For this review, take the finished solid that the model builds, in its own axes (mm). Coordinates: 2 decimals unless noted, no trailing zeros. Write each loop counter-clockwise with the first axis right and the second up, starting at its lowest first coordinate (ties: lowest second). Pieces come first, ordered by that corner, then holes.
```python
from build123d import *

# Parameters (mm, degrees)
CROQUIS1_R              = 3
CROQUIS1_R_2            = 4
SALIENTE_EXTRUIR1_DEPTH = 3


with BuildPart() as part:
    # Croquis1 → Saliente-Extruir1 (new body)
    with BuildSketch(Plane(origin=(0, 0, 0), x_dir=(1, 0, 0), z_dir=(0, 1, 0))):
        Polygon((17, 27.5), (0, 27.5), (-17, 27.5), (-17, 30.5), (-23.75, 30.5), (-30.5, 30.5), (-30.5, 23.75), (-40.5, 23.75), (-40.5, 8), (-37.5, 8), (-37.5, 0), (-37.5, -8), (-40.5, -8), (-40.5, -23.75), (-30.5, -23.75), (-30.5, -30.5), (-23.75, -30.5), (-17, -30.5), (-17, -27.5), (0, -27.5), (17, -27.5), (17, -30.5), (23.75, -30.5), (30.5, -30.5), (30.5, -23.75), (40.5, -23.75), (40.5, -8), (37.5, -8), (37.5, 0), (37.5, 8), (40.5, 8), (40.5, 23.75), (30.5, 23.75), (30.5, 30.5), (23.75, 30.5), (17, 30.5), align=None)
        Polygon((30.5, 17), (30.5, -17), (27.5, -17), (27.5, 0), (27.5, 17), align=None, mode=Mode.SUBTRACT)
        Polygon((-27.5, 17), (-27.5, 0), (-27.5, -17), (-30.5, -17), (-30.5, 17), align=None, mode=Mode.SUBTRACT)
        with Locations(Location((0, 0, 0), (0, 0, 270))):
            Circle(CROQUIS1_R, mode=Mode.SUBTRACT)
        with Locations(Location((18.5, 0, 0), (0, 0, 270))):
            Circle(CROQUIS1_R_2, mode=Mode.SUBTRACT)
    extrude(amount=SALIENTE_EXTRUIR1_DEPTH)


solid = part.part
```
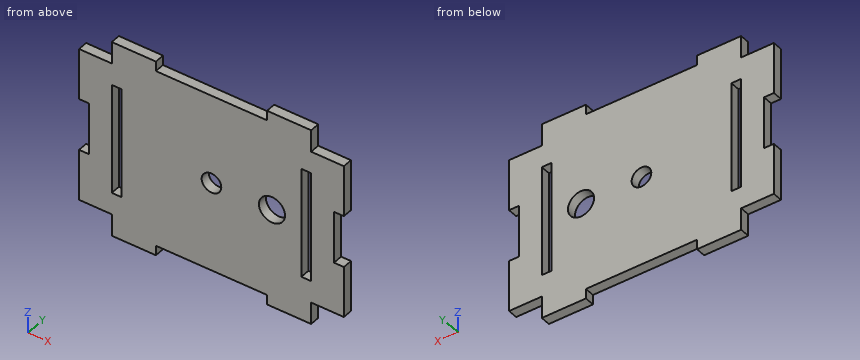
Q1. For probe 1 along X at (y, z) = (1.3, -10); probe 2 along X at (y, z) = (1.4, 0); probe 3 along X at (y, z) = (0.45, -3.5), list the stretches that pass through material, from the lowest coordinate up.
Ans:
probe 1: x = -40.5 to -30.5, -27.5 to 27.5, 30.5 to 40.5
probe 2: x = -37.5 to -30.5, -27.5 to -3, 3 to 14.5, 22.5 to 27.5, 30.5 to 37.5
probe 3: x = -37.5 to -30.5, -27.5 to 16.56, 20.44 to 27.5, 30.5 to 37.5
Q2. Add section A-A (z = 5.5). State the section outline as (x, y) points, then the cut area to 3 significant figures.
Ans:
outline: (-37.5, 0) - (-30.5, 0) - (-30.5, 3) - (-37.5, 3) - close; (-27.5, 0) - (27.5, 0) - (27.5, 3) - (-27.5, 3) - close; (30.5, 0) - (37.5, 0) - (37.5, 3) - (30.5, 3) - close
area: 207 mm2
Q3. Add section C-C (y = 1.05). Give the number of separate pieces and of enclosed holes in the cut face, then the cut area to 3 significant figures.
Ans:
separate pieces: 1
enclosed holes: 4
area: 4,090 mm2
Q4. Add section D-D (z = -10). State the section outline as (x, y) points, then the cut area to 3 significant figures.
Ans:
outline: (-40.5, 0) - (-30.5, 0) - (-30.5, 3) - (-40.5, 3) - close; (-27.5, 0) - (27.5, 0) - (27.5, 3) - (-27.5, 3) - close; (30.5, 0) - (40.5, 0) - (40.5, 3) - (30.5, 3) - close
area: 225 mm2
Q5. Add section B-B (x = 18.5). State the section outline as (y, z) points.
Ans:
outline: (0, -30.5) - (3, -30.5) - (3, -4) - (0, -4) - close; (0, 4) - (3, 4) - (3, 30.5) - (0, 30.5) - close
Q6. Clearance check with flat-ended pins moving along their axes: pin 1 Ø1.5 at (y, z) = (1, -28) entering from +X; pin 2 Ø1.5 at (y, z) = (2, -28) entering from -X. State where each tip first meets the part, or that it passes through.
Ans:
pin 1: stops at x = 30.5
pin 2: stops at x = -30.5
